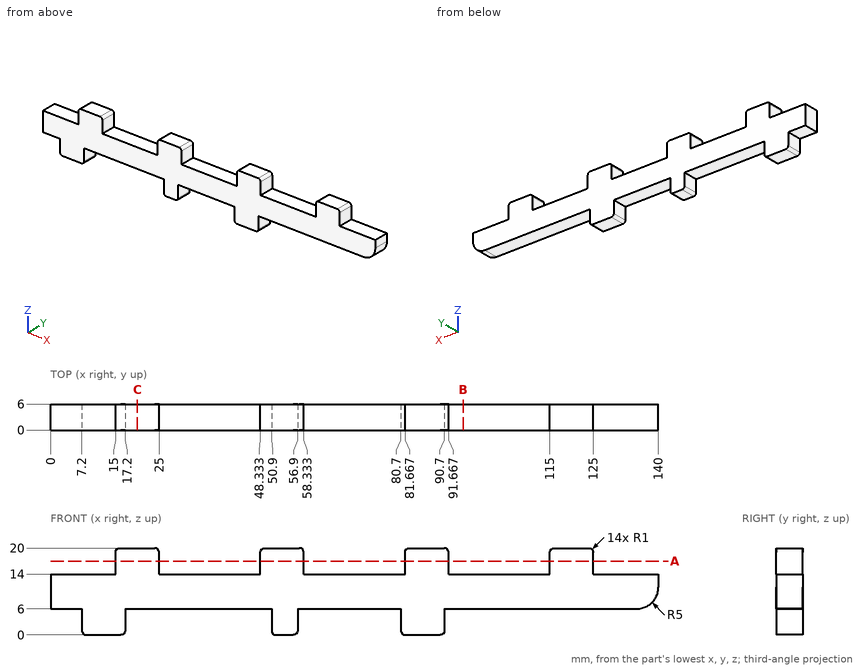
Print and shaded views of the part. All mm, measured from the part's lowest x, y and z. Coordinates: 2 decimals unless noted, no trailing zeros. Loops run counter-clockwise (first coordinate to the right, second up) from the corner with the lowest first, then second, coordinate; pieces in that order, holes last. Notation, with made-up numbers: (-7, -7.75) -> (49, -7.75) arc R6 ccw to (49, -2.75) -> close; hole circle Ø11 at (-6, -13). An arc over 180 degrees is marked (long way). Use one line per item in the form item = value. Start each with the question number.
(1) Cut at C-C on x = 20. Give the cut face in (y, z), and give its area (3 significant figures).
(2) Probe probe 1 along X at (y, z) = (5.35, 2.75); probe 2 along X at (y, z) = (2.65, 16.75); probe 3 along Z at (x, y) = (132, 0.45). List the from-to ranges inside material, lowest first. Write a range as from..to.
(3) Flat gauge pins, fed straight in: pin 1 (2.5 mm diameter, centred on y = 4, z = 16.5, fed in from +X); pin 2 (2.5 mm diameter, centred on y = 3.5, z = 15.5, fed in from -X); pin 3 (10 mm diameter, centred on x = 106.5, z = 8.5, fed in from -Y); pin 4 (1.8 mm diameter, centred on x = 131, y = 4.5, fed in from +Z). Where does each tip first touch, or does it go through?
(4) Cut at A-A on z = 17. Give the cut face in (x, y), and give its area (3 significant figures).
(5) Cut at B-B on x = 95. Give the cut face in (y, z), and give its area (3 significant figures).
Values:
q1.outline = (0, 6) -> (6, 6) -> (6, 20) -> (0, 20) -> close
q1.area = 84.0 mm2
q2.probe_1 = 7.2..17.2, 50.9..56.9, 80.7..90.7
q2.probe_2 = 15..25, 48.33..58.33, 81.67..91.67, 115..125
q2.probe_3 = 6..14
q3.pin_1 = 125
q3.pin_2 = 15
q3.pin_3 = 0
q3.pin_4 = 14
q4.outline = (15, 0) -> (25, 0) -> (25, 6) -> (15, 6) -> close; (48.33, 0) -> (58.33, 0) -> (58.33, 6) -> (48.33, 6) -> close; (81.67, 0) -> (91.67, 0) -> (91.67, 6) -> (81.67, 6) -> close; (115, 0) -> (125, 0) -> (125, 6) -> (115, 6) -> close
q4.area = 240 mm2
q5.outline = (0, 6) -> (6, 6) -> (6, 14) -> (0, 14) -> close
q5.area = 48.0 mm2
